Can you work these out from the drawing? Everything is in mm from the part's minimum corner. A direction names the side the tool comes from. Give positions to 0.01 mm unless a question says otherwise; leave off trailing zeros. Order: outer loops, then holes, each group sorted by start corner. A loop starts at its lowest first (then second) coordinate and runs counter-clockwise, first axis right, second up. Notation, with made-up numbers: (4, 80) -> (59, 80) arc R17 ccw to (59, 113) -> close; hole circle Ø7 at (-9, 42). An arc over 180 degrees is marked (long way). One line per item, written item: value.
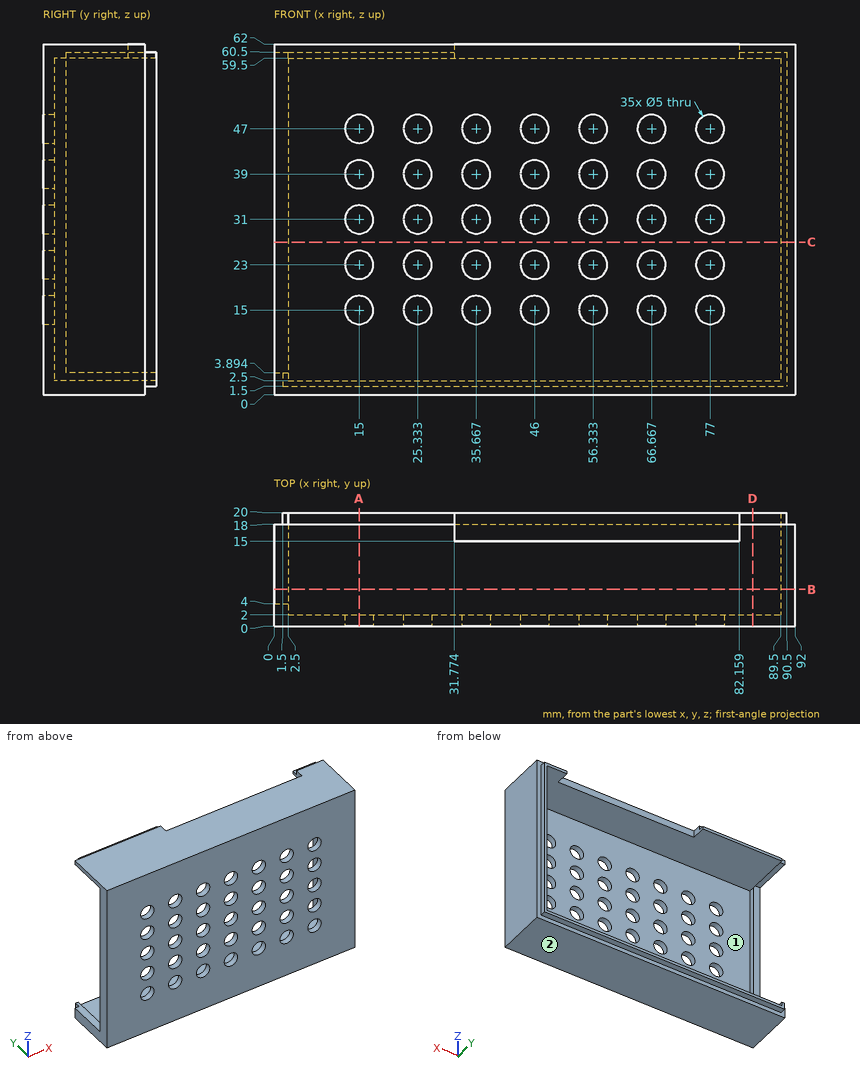
1) Suppose I cut it at C-C, the plane z = 27. Write out the boundary of the cut face in (x, y), then the cut area to 3 significant figures.
Answer below:
outline: (0, 0) -> (92, 0) -> (92, 18) -> (90.5, 18) -> (90.5, 20) -> (89.5, 20) -> (89.5, 2) -> (2.5, 2) -> (2.5, 4) -> (0, 4) -> close
area: 231 mm2
2) Suppose I cut it at B-B, the plane y = 6.5. Write out the boundary of the cut face in (x, z) (1 decimal).
Answer below:
outline: (0, 0) -> (92, 0) -> (92, 62) -> (0, 62) -> (0, 60.5) -> (2.5, 60.5) -> (2.5, 59.5) -> (89.5, 59.5) -> (89.5, 2.5) -> (2.5, 2.5) -> (2.5, 3.9) -> (0, 3.9) -> close
3) Suppose I cut it at A-A, the plane x = 15. State how many separate pieces and enclosed holes the cut face has, then the cut area to 3 significant figures.
Answer below:
separate pieces: 6
enclosed holes: 0
area: 158 mm2
4) Suppose I cut it at D-D, the plane x = 84.5. Write out the boundary of the cut face in (y, z), then the cut area to 3 significant figures.
Answer below:
outline: (0, 0) -> (18, 0) -> (18, 1.5) -> (20, 1.5) -> (20, 2.5) -> (2, 2.5) -> (2, 59.5) -> (20, 59.5) -> (20, 60.5) -> (18, 60.5) -> (18, 62) -> (0, 62) -> close
area: 208 mm2
5) For the marked faces 1 and 2, which set-ups out of +Z, -Z, +X, -X, +Y, -Y let a thin tool reach every point of the face, with its end or its side?
Answer below:
face 1: +Y
face 2: -Z, +X, -X, +Y, -Y
6) For P1, Ø4, axis at x = 56.33, z = 15, coming from the +Y side; P2, Ø5, axis at y = 15, z = 21.5, coming from the -X side; P3, Ø1.6, axis at x = 22.5, z = 61.5, coming from the +Y side; P4, Ø5, axis at x = 18.5, z = 52.5, coming from the +Y side, each with a flat end and sliding along its axis, tell me the tip position at first contact or that it passes through.
Answer below:
P1: passes through
P2: stops at x = 89.5
P3: stops at y = 18
P4: stops at y = 2
7) If I drill on line 1 along Z through (x, y) = (77, 1.4); line 2 along Z through (x, y) = (81.5, 13.5); line 3 along Y through (x, z) = (17.5, 19), over which ranges is the centre line in solid material (lowest first)?
Answer below:
line 1: z = 0 to 12.5, 17.5 to 20.5, 25.5 to 28.5, 33.5 to 36.5, 41.5 to 44.5, 49.5 to 62
line 2: z = 0 to 2.5, 59.5 to 62
line 3: y = 0 to 2
